Model file for the job. Use its own axes, mm. A direction names the side the tool comes from. Give positions to 0.01 mm unless a question says otherwise; leave off trailing zeros. Order: outer loops, then holes, each group sorted by start corner. A loop starts at its lowest first (then second) coordinate and runs counter-clockwise, first axis right, second up. Notation, with made-up numbers: (35.25, 26.25) - (43.25, 26.25) arc R18 cw to (43.25, 39.25) - close; hole circle Ø5 at (53, 76.25). An arc over 180 degrees is marked (long way). Return JSON: item names as keys, results as strings. Group by question number.
from build123d import *

# Parameters (mm, degrees)
F1_DEPTH  = 41.5
F2_R      = 0.45
F3_DEPTH  = 3.6
F1_FACE_W = 83
F1_FACE_H = 3
F4_DEPTH  = 3


with BuildPart() as f1:
    # F0 (on Right) → F1 (new body, symmetric)
    with BuildSketch(Plane.YZ):
        Polygon((0, 2.598076), (-1.5, 0), (1.5, 0), align=None)
    extrude(amount=F1_DEPTH, both=True)

    # F2 (on Top) → F3 (join)
    with BuildSketch(Plane.XY):
        with Locations((-32, 0)):
            Circle(F2_R)
        with Locations((-24, 0)):
            Circle(F2_R)
        with Locations((-16, 0)):
            Circle(F2_R)
        with Locations((-8, 0)):
            Circle(F2_R)
        Circle(F2_R)
        with Locations((8, 0)):
            Circle(F2_R)
        with Locations((16, 0)):
            Circle(F2_R)
        with Locations((24, 0)):
            Circle(F2_R)
        with Locations((32, 0)):
            Circle(F2_R)
    extrude(amount=F3_DEPTH)

    # F1_face (on face) → F4 (join)
    with BuildSketch(Plane(origin=(0, 0, 0), x_dir=(1, 0, 0), z_dir=(0, 0, -1))):
        Rectangle(F1_FACE_W, F1_FACE_H)
    extrude(amount=F4_DEPTH)


solid = f1.part
(1) Pull direction X, two halves, no side cores. Call faces 3 (the face through (41.5, 0, -1)), 4 (the face through (-1, -1.5, -1)), 5 (the face through (-41.5, 0, -1)), 6 (the face through (0.58, 0.76, 1.28)): released by +X, released by -X, zero draft, split by the parting line, or undercut.
(2) Slice it at B-B (z = 1). Give the cut face in (x, y).
(3) Drop a flat-ended pin along its axis: pin 1 Ø1 at (x, y) = (19.5, 0) entering from +Z. Give the stop position or say it passes through.
(4) Slice it at C-C (y = 1). Give the cut face in (x, z), and give its area (3 significant figures).
(5) Drill centre lines: L1, parallel to Z at x = -3, y = -0.3; L2, parallel to Z at x = 15, y = -1.1; L3, parallel to Y at x = -9, z = 2.25. Where is each one in solid material? Low to high.
(6) Slice it at A-A (x = -18). Give the cut face in (y, z), and give its area (3 significant figures).
(7) 3-axis set-ups, long thin cutter, end or side, ignore diameter. For faces 1 (the face through (0.58, -0.74, 1.32)), 2 (the face through (-1, 0, -3)): which of +Z, -Z, +X, -X, +Y, -Y reach the whole face in a straight line?
Result set:
{
 "1": {"face 3": "released by +X", "face 4": "zero draft", "face 5": "released by -X", "face 6": "undercut"},
 "2": {"outline": "(-41.5, -0.92) - (41.5, -0.92) - (41.5, 0.92) - (-41.5, 0.92) - close"},
 "3": {"pin 1": "stops at z = 2.6"},
 "4": {"outline": "(-41.5, -3) - (41.5, -3) - (41.5, 0.87) - (-41.5, 0.87) - close", "area": "321 mm²"},
 "5": {"L1": "z = -3 to 2.08", "L2": "z = -3 to 0.69", "L3": "y = -0.2 to 0.2"},
 "6": {"outline": "(-1.5, -3) - (1.5, -3) - (1.5, 0) - (0, 2.6) - (-1.5, 0) - close", "area": "12.9 mm²"},
 "7": {"face 1": "+Z, -Y", "face 2": "-Z, +X, -X, +Y, -Y"}
}
